Geometry check sheet. Reference: the model listing, model coordinates, mm. A direction names the side the tool comes from. Give positions to 0.01 mm unless a question says otherwise; leave off trailing zeros. Order: outer loops, then holes, each group sorted by start corner. A loop starts at its lowest first (then second) coordinate and runs counter-clockwise, first axis right, second up.
from build123d import *

# Parameters (mm, degrees)
SKETCH1_W           = 30
SKETCH1_H           = 10
SKETCH1_R           = 3
BOSS_EXTRUDE1_DEPTH = 5
SKETCH1_2_R         = 3
BOSS_EXTRUDE2_DEPTH = 20


with BuildPart() as part:
    # Sketch1 → Boss-Extrude1 (new body)
    with BuildSketch(Plane(origin=(0, 0, 0), x_dir=(1, 0, 0), z_dir=(0, 1, 0))):
        with Locations((11.25, 0)):
            Rectangle(SKETCH1_W, SKETCH1_H)
        with Locations(Location((0, 0, 0), (0, 0, 270))):
            Circle(SKETCH1_R, mode=Mode.SUBTRACT)
        with Locations(Location((22.5, 0, 0), (0, 0, 270))):
            Circle(SKETCH1_R, mode=Mode.SUBTRACT)
    extrude(amount=BOSS_EXTRUDE1_DEPTH)

    # Sketch1_2 → Boss-Extrude2 (add)
    with BuildSketch(Plane(origin=(0, 0, 0), x_dir=(1, 0, 0), z_dir=(0, 1, 0))):
        with Locations(Location((0, 0, 0), (0, 0, 270))):
            Circle(SKETCH1_2_R)
        with Locations(Location((22.5, 0, 0), (0, 0, 270))):
            Circle(SKETCH1_2_R)
    extrude(amount=BOSS_EXTRUDE2_DEPTH)


solid = part.part
Item 1: Sectioned sample at A-A (x = 0). Enter the section's corners in (y, z), and give its area (3 significant figures).
Reported:
outline: (0, -5) - (5, -5) - (5, -3) - (20, -3) - (20, 3) - (5, 3) - (5, 5) - (0, 5) - close
area: 140 mm2
Item 2: Set-up check for faces 4 (the cylindrical face through (0.9, 12.4, 2.86)), 5 (the flat face through (11, 0, 0)): record each of +Z, -Z, +X, -X, +Y, -Y from which the full face is reachable in a straight line by a thin tool's end or side.
Reported:
face 4: +Y
face 5: +Z, -Z, +X, -X, -Y
Item 3: Sectioned sample at C-C (y = 11.75). Enter the section's corners in (x, z), and give its area (3 significant figures).
Reported:
outline: circle Ø6 at (0, 0); circle Ø6 at (22.5, 0)
area: 56.5 mm2
Item 4: Draft check along X on faces 1 (the flat face through (11, 2, -5)), 2 (the flat face through (11, 5, 0)), 3 (the flat face through (26.25, 2, 0)). Enter one of: released by +X, released by -X, zero draft, split by the parting line, or undercut.
Reported:
face 1: zero draft
face 2: undercut
face 3: released by +X
Item 5: Scan lines: L1, parallel to X at y = 12, z = 2.75; L2, parallel to Y at x = 19, z = -0.75; L3, parallel to X at y = 15.75, z = 2.5. Record each from-to range of solid material in increasing order.
Reported:
L1: x = -1.2 to 1.2, 21.3 to 23.7
L2: y = 0 to 5
L3: x = -1.66 to 1.66, 20.84 to 24.16
Item 6: Sectioned sample at B-B (z = 0). Enter the section's corners in (x, y), and give its area (3 significant figures).
Reported:
outline: (-3.75, 0) - (26.25, 0) - (26.25, 5) - (25.5, 5) - (25.5, 20) - (19.5, 20) - (19.5, 5) - (3, 5) - (3, 20) - (-3, 20) - (-3, 5) - (-3.75, 5) - close
area: 330 mm2
Item 7: Sectioned sample at D-D (z = -2.5). Enter the section's corners in (x, y), and give its area (3 significant figures).
Reported:
outline: (-3.75, 0) - (26.25, 0) - (26.25, 5) - (24.16, 5) - (24.16, 20) - (20.84, 20) - (20.84, 5) - (1.66, 5) - (1.66, 20) - (-1.66, 20) - (-1.66, 5) - (-3.75, 5) - close
area: 249 mm2
Item 8: Gauge pin test, flat ends, axial feed: pin 1 (6 mm diameter, centred on y = 16.5, z = 2, fed in from +X); pin 2 (2 mm diameter, centred on y = 6.5, z = -2, fed in from -X); pin 3 (1.5 mm diameter, centred on y = 8.5, z = 2, fed in from -X). Record the tip position at first contact, or that the pin passes through.
Reported:
pin 1: stops at x = 25.5
pin 2: stops at x = -2.83
pin 3: stops at x = -2.73
